For this review, take the finished solid that the model builds, in its own axes (mm). Face numbers are marked on the shaded views. A direction names the side the tool comes from. Give positions to 0.01 mm unless a question says otherwise; leave off trailing zeros. Write each loop counter-clockwise with the first axis right and the second up, starting at its lowest first coordinate (ties: lowest second). Pieces come first, ordered by that corner, then holes.
1) For P1, Ø3, axis at x = 15.91, y = 15.91, coming from the -Z side; P2, Ø1, axis at x = 6, z = -4.5, coming from the -Y side; P3, Ø2, axis at y = -0.5, z = -11, coming from the -X side; P4, Ø6.5, axis at x = -0.5, y = 3, coming from the -Z side, all flat-tipped, find the tip position at first contact; note any pin that passes through.
2) We need section A-A on z = 2. Give the boundary of the cut face in (x, y).
3) We need section B-B on x = 0. Give the boundary of the cut face in (y, z), and give its area (3 significant figures).
4) Machinability: for the marked faces 1 and 2, which of the approach directions +Z, -Z, +X, -X, +Y, -Y give a long, thin tool a straight path to every point of the face, cutting with its end or side? Answer none if there is none.
5) We need section D-D on z = -20. Give the boundary of the cut face in (x, y), and give its area (3 significant figures).
6) We need section C-C on y = -3.5. Give the boundary of the cut face in (x, z), and give its area (3 significant figures).
7) Wall thickness on line 1 along Y through (x, z) = (0, -1); line 2 along X through (y, z) = (15.5, 4.5); line 3 along Z through (x, y) = (8, -9.5): over which ranges is each line inside the solid? List them lowest first.
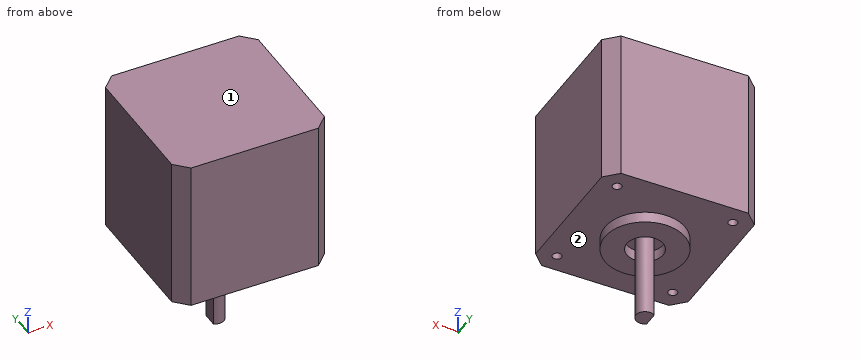
from build123d import *

# Parameters (mm, degrees)
SALIENTE_EXTRUIR1_DEPTH = 42
CROQUIS2_R              = 11
CROQUIS2_R_2            = 5
SALIENTE_EXTRUIR3_DEPTH = 3
SALIENTE_EXTRUIR4_DEPTH = 24
CROQUIS7_R              = 1.25
CORTAR_EXTRUIR2_DEPTH   = 15


with BuildPart() as part:
    # Croquis1 → Saliente-Extruir1 (new body)
    with BuildSketch(Plane.XY):
        Polygon((-17.5, -21), (17.5, -21), (21, -17.5), (21, 17.5), (17.5, 21), (-17.5, 21), (-21, 17.5), (-21, -17.5), align=None)
    extrude(amount=SALIENTE_EXTRUIR1_DEPTH)

    # Croquis2 → Saliente-Extruir3 (add)
    with BuildSketch(Plane(origin=(0, 0, 0), x_dir=(-1, 0, 0), z_dir=(0, 0, -1))):
        with Locations(Location((0, 0, 0), (0, 0, 180))):
            Circle(CROQUIS2_R)
        Circle(CROQUIS2_R_2, mode=Mode.SUBTRACT)
    extrude(amount=SALIENTE_EXTRUIR3_DEPTH)

    # Croquis3 → Saliente-Extruir4 (add)
    with BuildSketch(Plane(origin=(0, 0, 0), x_dir=(-1, 0, 0), z_dir=(0, 0, -1))):
        with BuildLine():
            Line((1.5, 0), (-2.5, 0))
            ThreePointArc((-2.5, 0), (-1.118033989, -2.236067977), (1.5, -2))
            Line((1.5, -2), (1.5, 0))
        make_face()
        with BuildLine():
            ThreePointArc((1.5, 2), (-1.118033989, 2.236067977), (-2.5, 0))
            Line((-2.5, 0), (1.5, 0))
            Line((1.5, 0), (1.5, 2))
        make_face()
    extrude(amount=SALIENTE_EXTRUIR4_DEPTH)

    # Croquis7 → Cortar-Extruir2 (cut)
    with BuildSketch(Plane(origin=(0, 0, 0), x_dir=(-1, 0, 0), z_dir=(0, 0, -1))):
        with Locations((-15.909902577, 15.909902577)):
            Circle(CROQUIS7_R)
        with Locations((-15.909902577, -15.909902577)):
            Circle(CROQUIS7_R)
        with Locations((15.909902577, -15.909902577)):
            Circle(CROQUIS7_R)
        with Locations((15.909902577, 15.909902577)):
            Circle(CROQUIS7_R)
    extrude(amount=-CORTAR_EXTRUIR2_DEPTH, mode=Mode.SUBTRACT)


solid = part.part
Results list:
1. P1: stops at z = 0
1. P2: passes through
1. P3: stops at x = -1.5
1. P4: stops at z = -24
2. outline: (-21, -17.5) - (-17.5, -21) - (17.5, -21) - (21, -17.5) - (21, 17.5) - (17.5, 21) - (-17.5, 21) - (-21, 17.5) - close; hole circle Ø2.5 at (-15.91, -15.91); hole circle Ø2.5 at (-15.91, 15.91); hole circle Ø2.5 at (15.91, -15.91); hole circle Ø2.5 at (15.91, 15.91)
3. outline: (-21, 0) - (-11, 0) - (-11, -3) - (-5, -3) - (-5, 0) - (-2.5, 0) - (-2.5, -24) - (2.5, -24) - (2.5, 0) - (5, 0) - (5, -3) - (11, -3) - (11, 0) - (21, 0) - (21, 42) - (-21, 42) - close
3. area: 1,920 mm2
4. face 1: +Z, +X, -X, +Y, -Y
4. face 2: -Z
5. outline: (-1.5, -2) arc R2.5 ccw (long way) to (-1.5, 2) - close
5. area: 16.8 mm2
6. outline: (-21, 0) - (-10.43, 0) - (-10.43, -3) - (-3.57, -3) - (-3.57, 0) - (3.57, 0) - (3.57, -3) - (10.43, -3) - (10.43, 0) - (21, 0) - (21, 42) - (-21, 42) - close
6. area: 1,810 mm2
7. line 1: y = -11 to -5, -2.5 to 2.5, 5 to 11
7. line 2: x = -21 to -17.09, -14.73 to 14.73, 17.09 to 21
7. line 3: z = 0 to 42
